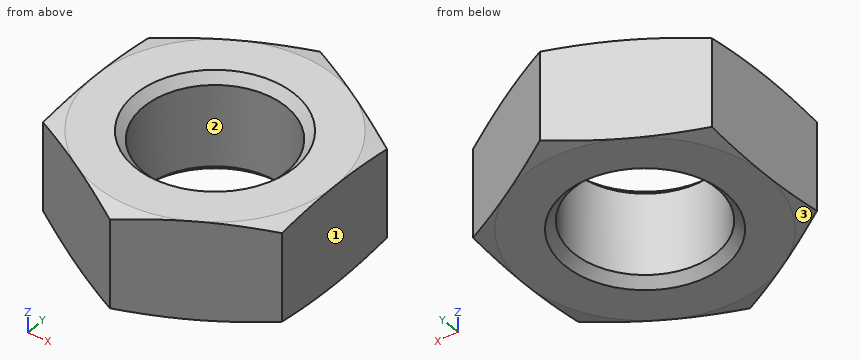
Autodesk Inventor part; units mm, degrees
ref_plane "NUT_XY" through (0, 0, 0) normal (0, 0, 1) x (1, 0, 0)
ref_plane "NUT_YZ" through (0, 0, 0) normal (1, 0, 0) x (0, 1, 0)
ref_plane "NUT_ZX" through (0, 0, 0) normal (0, 1, 0) x (0, 0, 1)
sketch "Sketch_8" plane through (0, 0, 0) normal (1, 0, 0) x (0, 1, 0)
  line L0 (0, -7.874) -> (0, 0)
  line L1 (0, 0) -> (9.525, 0)
  line L2 (9.525, 0) -> (11.43, -0.5104)
  line L3 (11.43, -0.5104) -> (11.43, -7.3636)
  line L4 (11.43, -7.3636) -> (9.525, -7.874)
  line L5 (9.525, -7.874) -> (0, -7.874)
  line L6 (0, -7.874) -> (0, 0)
sketch "Sketch_10" plane through (0, 0, 0) normal (0, 0, 1) x (1, 0, 0)
  line L0 (-19.05, 19.05) -> (-19.05, -19.05)
  line L1 (-19.05, -19.05) -> (19.05, -19.05)
  line L2 (19.05, -19.05) -> (19.05, 19.05)
  line L3 (19.05, 19.05) -> (-19.05, 19.05)
  line L4 (-9.525, 5.4993) -> (-9.525, -5.4993)
  line L5 (-9.525, -5.4993) -> (0, -10.9985)
  line L6 (0, -10.9985) -> (9.525, -5.4993)
  line L7 (9.525, -5.4993) -> (9.525, 5.4993)
  line L8 (9.525, 5.4993) -> (0, 10.9985)
  line L9 (0, 10.9985) -> (-9.525, 5.4993)
revolve "Revolution1" add sketch "Sketch_8" angle 360 about axis through (0, 0, -7.874) along (0, 0, -1)
extrude "Extrusion1" cut sketch "Sketch_10" against normal blind 7.874
sketch "Sketch_11" plane through (0, 0, 0) normal (1, 0, 0) x (0, 1, 0)
  line L0 (0, -7.874) -> (0, 0)
  line L1 (0, 0) -> (6.35, 0)
  line L2 (6.35, 0) -> (5.6629, -0.6871)
  line L3 (5.6629, -0.6871) -> (5.6629, -7.1869)
  line L4 (5.6629, -7.1869) -> (6.35, -7.874)
  line L5 (6.35, -7.874) -> (0, -7.874)
  line L6 (0, -7.874) -> (0, 0)
revolve "Revolution2" cut sketch "Sketch_11" angle 360 about axis through (0, 0, -7.874) along (0, 0, -1)
thread "Thread1"
ref_plane "NUT_XY" through (0, 0, 0) normal (0, 0, 1) x (1, 0, 0)
ref_plane "NUT_YZ" through (0, 0, 0) normal (1, 0, 0) x (0, 1, 0)
ref_plane "NUT_ZX" through (0, 0, 0) normal (0, 1, 0) x (0, 0, 1)
ref_plane "a1_XY" through (-9.525, 9.525, 0) normal (0, 0, 1) x (1, 0, 0)
ref_plane "a1_YZ" through (-9.525, 9.525, 0) normal (1, 0, 0) x (0, 1, 0)
ref_plane "a1_ZX" through (-9.525, 9.525, 0) normal (0, 1, 0) x (0, 0, 1)
ref_plane "a2_XY" through (9.525, 9.525, 0) normal (0, 0, 1) x (1, 0, 0)
ref_plane "a2_YZ" through (9.525, 9.525, 0) normal (1, 0, 0) x (0, 1, 0)
ref_plane "a2_ZX" through (9.525, 9.525, 0) normal (0, 1, 0) x (0, 0, 1)
ref_plane "b1_XY" through (0, 9.525, 0) normal (1, 0, 0) x (0, 0, -1)
ref_plane "b1_YZ" through (0, 9.525, 0) normal (0, 0, -1) x (0, 1, 0)
ref_plane "b1_ZX" through (0, 9.525, 0) normal (0, 1, 0) x (1, 0, 0)
ref_plane "b2_XY" through (0, 9.525, -7.874) normal (1, 0, 0) x (0, 0, -1)
ref_plane "b2_YZ" through (0, 9.525, -7.874) normal (0, 0, -1) x (0, 1, 0)
ref_plane "b2_ZX" through (0, 9.525, -7.874) normal (0, 1, 0) x (1, 0, 0)
ref_plane "e_XY" through (0, 0, -7.874) normal (1, 0, 0) x (0, 0, -1)
ref_plane "e_YZ" through (0, 0, -7.874) normal (0, 0, -1) x (0, 1, 0)
ref_plane "e_ZX" through (0, 0, -7.874) normal (0, 1, 0) x (1, 0, 0)
ref_plane "th1_XY" through (0, 6.35, -7.874) normal (1, 0, 0) x (0, 0, -1)
ref_plane "th1_YZ" through (0, 6.35, -7.874) normal (0, 0, -1) x (0, 1, 0)
ref_plane "th1_ZX" through (0, 6.35, -7.874) normal (0, 1, 0) x (1, 0, 0)
ref_plane "th2_XY" through (0, -6.35, -7.874) normal (1, 0, 0) x (0, 0, -1)
ref_plane "th2_YZ" through (0, -6.35, -7.874) normal (0, 0, -1) x (0, 1, 0)
ref_plane "th2_ZX" through (0, -6.35, -7.874) normal (0, 1, 0) x (1, 0, 0)
ref_plane "ol1_XY" through (0, 0, -9.525) normal (0, 1, 0) x (1, 0, 0)
ref_plane "ol1_YZ" through (0, 0, -9.525) normal (1, 0, 0) x (0, 0, -1)
ref_plane "ol1_ZX" through (0, 0, -9.525) normal (0, 0, -1) x (0, 1, 0)
ref_plane "ol2_XY" through (7.874, 0, -9.525) normal (0, 1, 0) x (1, 0, 0)
ref_plane "ol2_YZ" through (7.874, 0, -9.525) normal (1, 0, 0) x (0, 0, -1)
ref_plane "ol2_ZX" through (7.874, 0, -9.525) normal (0, 0, -1) x (0, 1, 0)
properties part number "D-98"
Geometry: final body of the model. Coordinates: model frame, mm. Face numbers are marked on the shaded views. Give positions to 0.01 mm unless a question says otherwise; leave off trailing zeros. Write each loop counter-clockwise with the first axis right and the second up, starting at its lowest first coordinate (ties: lowest second). Pieces come first, ordered by that corner, then holes. Notation, with made-up numbers: (-22.75, 29.25) -> (14.25, 29.25) arc R6 cw to (14.25, 35.25) -> close; hole circle Ø3 at (7, -3). An arc over 180 degrees is marked (long way). Answer in a Markdown table with one row per item.
(1) Ray query, line 1 along X through (y, z) = (0, -2.75) (3 decimals); line 2 along Y through (x, z) = (4, -5.25); line 3 along Y through (x, z) = (3, -6). Return the intervals inside material, ascending. Write a range as [from, to].
Answers below:
| item | result |
|---|---|
| line 1 | [-9.525, -5.663], [5.663, 9.525] |
| line 2 | [-8.69, -4.01], [4.01, 8.69] |
| line 3 | [-9.27, -4.8], [4.8, 9.27] |
(2) Pin query (flat end, axial travel): pin 1 (3 mm diameter, centred on x = 5, z = -1.5, fed in from -Y). Return the tip coordinate at first contact, or that it passes through.
Answers below:
| item | result |
|---|---|
| pin 1 | y = -8.98 |
(3) Section query A-A on z = -1. Return loops of the section in (x, y) (1 decimal).
Answers below:
| item | result |
|---|---|
| outline | (-9.5, -5.5) -> (0, -11) -> (9.5, -5.5) -> (9.5, 5.5) -> (0, 11) -> (-9.5, 5.5) -> close; hole circle Ø11.3 at (0, 0) |
(4) Draft query along X for the marked faces 1, 2 and 3. Return one class per face: +X half, -X half, draft (parallel to the pull), parting line (faces both ways), or undercut.
Answers below:
| item | result |
|---|---|
| face 1 | +X half |
| face 2 | undercut |
| face 3 | -X half |
